For this review, take the finished solid that the model builds, in its own axes (mm). Face numbers are marked on the shaded views. A direction names the side the tool comes from. Give positions to 0.01 mm unless a question says otherwise; leave off trailing zeros. Loops run counter-clockwise (first coordinate to the right, second up) from the corner with the lowest first, then second, coordinate; pieces in that order, holes last. Notation, with made-up numbers: (9, 85) -> (42, 85) arc R29 cw to (42, 107) -> close; hole circle Ø3 at (80.5, 74). An arc over 180 degrees is marked (long way). Answer as CSV lines item,"result". Start each with the question number.
Item 1: Add section A-A on x = -7. State the section outline as (y, z) points, plus the area to 3 significant figures.
Item 2: Clearance check with flat-ended pins moving along their axes: P1, Ø3, axis at y = 5.5, z = 35, coming from the -X side; P2, Ø6, axis at y = -5.5, z = 30, coming from the -X side; P3, Ø1.5, axis at y = -5.5, z = -8.5, coming from the -X side; P4, Ø6, axis at x = -154.328, z = 12.7, coming from the -Y side. State where each tip first meets the part, or that it passes through.
Item 3: Add section D-D on z = 21. State the section outline as (x, y) points.
Item 4: For L1, parallel to Z at x = -30.5, y = 6; L2, parallel to Z at x = -126.5, y = -6.25; L3, parallel to X at y = 7.75, z = 15, list the stretches that pass through material, from the lowest coordinate up. Write a range as from..to.
Item 5: Machinability: for the marked faces 5 and 6, which of the approach directions +Z, -Z, +X, -X, +Y, -Y give a long, thin tool a straight path to every point of the face, cutting with its end or side? Answer none if there is none.
Item 6: Add section C-C on x = -154. State the section outline as (y, z) points.
Item 7: Add section B-B on y = 0. State the section outline as (x, z) points.
Item 8: The part is to be moulded in two halves that separate along Z. For the marked faces 1, 2, 3 and 4, say which applies: +Z half, -Z half, draft (parallel to the pull), parting line (faces both ways), or undercut.
```python
from build123d import *

# Parameters (mm, degrees)
F0_R     = 5.122277
F1_DEPTH = 12.7


with BuildPart() as f1:
    # F0 (on Front) → F1 (new body, symmetric)
    with BuildSketch(Plane.XZ):
        with BuildLine():
            Line((-167.027999, 0), (-94.760983, 0))
            ThreePointArc((-94.760983, 0), (-85.513701, -3.994957), (-82.084134, -13.466491))
            ThreePointArc((-82.084134, -13.466491), (-78.112329, -21.947282), (-69.407286, -25.4))
            Line((-69.407286, -25.4), (17.726313, -25.4))
            Line((17.726313, -25.4), (17.726313, 0))
            Line((17.726313, 0), (-44.7079, 0))
            ThreePointArc((-44.7079, 0), (-53.688157, 3.719744), (-57.4079, 12.7))
            ThreePointArc((-57.4079, 12.7), (-53.688157, 21.680256), (-44.7079, 25.4))
            Line((-44.7079, 25.4), (18.7921, 25.4))
            Line((18.7921, 25.4), (18.7921, 50.8))
            Line((18.7921, 50.8), (-70.1079, 50.8))
            ThreePointArc((-70.1079, 50.8), (-79.088157, 47.080256), (-82.8079, 38.1))
            ThreePointArc((-82.8079, 38.1), (-86.527644, 29.119744), (-95.5079, 25.4))
            Line((-95.5079, 25.4), (-167.027999, 25.4))
            Line((-167.027999, 25.4), (-167.027999, 0))
        make_face()
        with Locations((-154.327999, 12.7)):
            Circle(F0_R, mode=Mode.SUBTRACT)
    extrude(amount=F1_DEPTH, both=True)


solid = f1.part
```
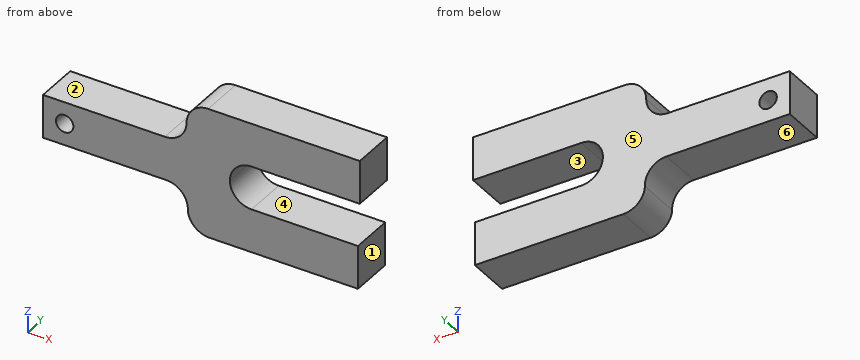
Computed values:
1,outline,"(-12.7, -25.4) -> (12.7, -25.4) -> (12.7, 0) -> (-12.7, 0) -> close; (-12.7, 25.4) -> (12.7, 25.4) -> (12.7, 50.8) -> (-12.7, 50.8) -> close"
1,area,"1,290 mm²"
2,P1,"x = -83.67"
2,P2,"x = -89.34"
2,P3,"x = -83.07"
2,P4,"through"
3,outline,"(-167.03, -12.7) -> (-54.32, -12.7) -> (-54.32, 12.7) -> (-167.03, 12.7) -> close"
4,L1,"-25.4..0, 25.4..50.8"
4,L2,"0..25.4"
4,L3,"-167.03..-158.9, -149.75..-57.2"
5,face 5,"+Z, -Z, +X, -X, +Y"
5,face 6,"-Z, -X, +Y, -Y"
6,outline,"(-12.7, 0) -> (12.7, 0) -> (12.7, 7.59) -> (-12.7, 7.59) -> close; (-12.7, 17.81) -> (12.7, 17.81) -> (12.7, 25.4) -> (-12.7, 25.4) -> close"
7,outline,"(-167.03, 0) -> (-94.76, 0) arc R12.7 cw to (-82.08, -13.47) arc R12.7 ccw to (-69.41, -25.4) -> (17.73, -25.4) -> (17.73, 0) -> (-44.71, 0) arc R12.7 cw to (-57.41, 12.7) arc R12.7 cw to (-44.71, 25.4) -> (18.79, 25.4) -> (18.79, 50.8) -> (-70.11, 50.8) arc R12.7 ccw to (-82.81, 38.1) arc R12.7 cw to (-95.51, 25.4) -> (-167.03, 25.4) -> close; hole circle Ø10.24 at (-154.33, 12.7)"
8,face 1,"draft"
8,face 2,"+Z half"
8,face 3,"undercut"
8,face 4,"undercut"
